Autodesk Inventor part; units mm, degrees
ref_plane "YZ Plane" through (0, 0, 0) normal (1, 0, 0) x (0, 1, 0)
ref_plane "XZ Plane" through (0, 0, 0) normal (0, 1, 0) x (-1, 0, 0)
ref_plane "XY Plane" through (0, 0, 0) normal (0, 0, 1) x (1, 0, 0)
sketch "Sketch1" plane through (0, 0, 0) normal (0, 1, 0) x (-1, 0, 0)
  circle A0 centre (0, 0) radius 52.5
  line L0 (0, 0) -> (52.5, 0)
  line L1 (52.5, 0) -> (0, 0)
  line L2 (52.5, 0) -> (0, 0)
  line L3 (0, 0) -> (-26.25, 0)
  line L4 (-26.25, 0) -> (-26.25, 45.4663)
  line L5 (52.5, 0) -> (-26.25, 45.4663)
  line L6 (-26.25, 0) -> (-26.25, -45.4663)
  line L7 (52.5, 0) -> (-26.25, -45.4663)
extrude "Extrusion1" add sketch "Sketch1" along normal blind 5 contours L7 L6 L3 L0 | L0 L3 L4 L5
sketch "Sketch5" plane through (0, 5, 0) normal (0, 1, 0) x (1, 0, 0)
  circle A0 centre (0, 0) radius 4.25
  dimension "d9" = 8.5
extrude "Extrusion3" cut sketch "Sketch5" against normal blind 2
sketch "Sketch6" plane through (0, 5, 0) normal (0, 1, 0) x (1, 0, 0)
  circle A0 centre (0, 0) radius 2.5
  dimension "d12" = 5
extrude "Extrusion4" add sketch "Sketch6" against normal blind 10
sketch "Sketch7" plane through (0, 5, 0) normal (0, 1, 0) x (1, 0, 0)
  circle A0 centre (0, 0) radius 4.25
  circle A1 centre (0, 0) radius 2.5
extrude "Extrusion5" cut sketch "Sketch7" against normal through all contours A1
sketch "Sketch8" plane through (0, 5, 0) normal (0, 1, 0) x (1, 0, 0)
  line L0 (-52.5, 0) -> (26.25, -45.4663)
  line L1 (-52.5, 0) -> (26.25, -45.4663)
  line L2 (26.25, 45.4663) -> (-52.5, 0)
  line L3 (26.25, -45.4663) -> (26.25, 45.4663)
  line L4 (26.25, 45.4663) -> (-52.5, 0)
  line L5 (26.25, -45.4663) -> (26.25, 45.4663)
  line L6 (26.25, 0) -> (23.75, 0)
  line L7 (-13.125, -22.7332) -> (-11.875, -20.5681)
  line L8 (-13.125, 22.7332) -> (-11.875, 20.5681)
  line L9 (-11.875, -20.5681) -> (-47.5, 0)
  line L10 (-47.5, 0) -> (-11.875, 20.5681)
  line L11 (23.75, 0) -> (23.75, 41.1362)
  line L12 (23.75, 41.1362) -> (-11.875, 20.5681)
  line L13 (23.75, 0) -> (23.75, -41.1362)
  line L14 (-11.875, -20.5681) -> (23.75, -41.1362)
  point P0 (0, 0)
  dimension "d17" = 2.5
  dimension "d18" = 2.5
extrude "Extrusion6" add sketch "Sketch8" along normal blind 40 contours L2 L8 L10 L9 L7 L0 | L7 L14 L13 L6 L3 L0 | L2 L3 L6 L11 L12 L8
fillet "Fillet1" radius 2.5 3 edges at (-11.875, 45, -20.5681) (23.75, 45, 0) (-11.875, 45, 20.5681)
properties part number "TrojkatP"
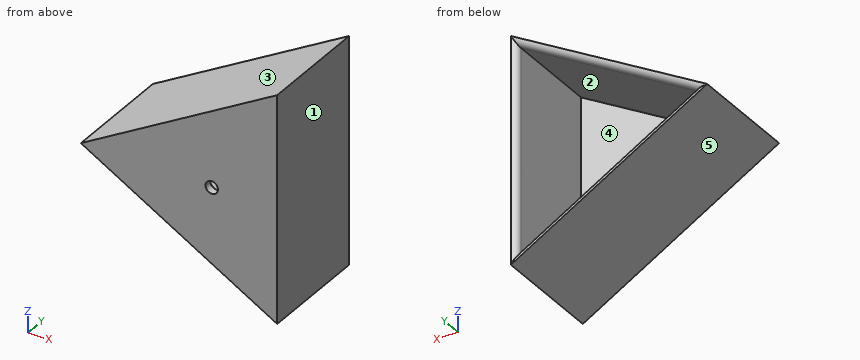
The listing builds one solid part. Answer for the finished solid, in the listing's coordinates (mm). Face numbers are marked on the shaded views. A direction names the side the tool comes from. Give positions to 0.01 mm unless a question says otherwise; leave off trailing zeros. Write each loop counter-clockwise with the first axis right and the second up, starting at its lowest first coordinate (ties: lowest second). Pieces come first, ordered by that corner, then holes.
1) Section A-A (y = 22.5) is taken. Write down the section's boundary in (x, z), and give its area (3 significant figures).
2) Given P1, Ø7, axis at x = -1, z = 2, coming from the +Y side; P2, Ø5, axis at x = -13.5, y = 40, coming from the -Z side; P3, Ø6, axis at y = 16.5, z = -7, coming from the -X side; P4, Ø3, axis at x = 0, z = 0, coming from the -Y side, each flat-ended and moving along its own axis, determine where each tip first touches the part or whether it passes through.
3) A tool of negligible diameter and unlimited length cuts with its end or side. For the marked faces 4 and 5, from which of +Z, -Z, +X, -X, +Y, -Y can it reach the whole face along a straight path? Write none if from no direction.
4) Find the intervals of material crossed by L1, parallel to Y at x = -1, z = -11.5; L2, parallel to Z at x = -8, y = 41.5; L3, parallel to Z at x = -3, y = 12.5, in increasing order.
5) For a pull along Z with two mould halves and no side action, classify the marked faces 1, 2 and 3 as pulls with the +Z half, pulls with the -Z half, needs draft (parallel to the pull), parting line crosses it, or undercut.
Response:
1. outline: (-52.5, 0) - (26.25, -45.47) - (26.25, 45.47) - close; hole (-47.5, 0) - (23.75, -41.14) - (23.75, 41.14) - close
1. area: 650 mm2
2. P1: stops at y = 5
2. P2: stops at z = -23.96
2. P3: stops at x = -45.57
2. P4: passes through
3. face 4: +Y
3. face 5: -Z, -X, +Y, -Y
4. L1: y = 0 to 5
4. L2: z = -25.69 to -22.81, 22.81 to 25.69
4. L3: z = -28.58 to -25.69, 25.69 to 28.58
5. face 1: needs draft
5. face 2: undercut
5. face 3: pulls with the +Z half
